The listing builds one solid part. Answer for the finished solid, in the listing's coordinates (mm). Face numbers are marked on the shaded views. Coordinates: 2 decimals unless noted, no trailing zeros. Write each loop counter-clockwise with the first axis right and the second up, starting at its lowest first coordinate (ties: lowest second). Pieces come first, ordered by that corner, then holes.
(1) Given P1, Ø4, axis at x = 2.5, y = -2, coming from the -Z side; P2, Ø1.5, axis at y = -5, z = 2.5, coming from the -X side, each flat-ended and moving along its own axis, determine where each tip first touches the part or whether it passes through.
(2) Straight lines are drawn through the part: line 1 (Y direction, x = 0, z = 1.25); line 2 (Y direction, x = -4, z = 0.25); line 3 (X direction, y = 0.5, z = 2.1). For each, find the intervals that lie inside material, in ascending order.
(3) The part is cut by section A-A on z = 1.25. Determine the outline of the cut face in (x, y), plus the area to 3 significant figures.
(4) The part is cut by section B-B on x = 0. Determine the outline of the cut face in (y, z).
(5) For a pull along Y with two mould halves and no side action, classify the marked faces 1, 2, 3 and 4 as +Y half, -Y half, draft (parallel to the pull), parting line (faces both ways), or undercut.
from build123d import *

# Parameters (mm, degrees)
SKIZZE2_W                            = 69.6667
SKIZZE2_H                            = 68.6667
SCHNITT_LINEAR_AUSTRAGEN1_DEPTH      = 10
SCHNITT_LINEAR_AUSTRAGEN1_DEPTH_BACK = 10


with BuildPart() as part:
    # Skizze1 → Rotation1 (revolve)
    with BuildSketch(Plane(origin=(0, 0, 0), x_dir=(0, 0, -1), z_dir=(1, 0, 0))):
        Polygon((-3, 6.5), (-3, 5), (-2.4585, 4.4585), (-0.5415, 4.4585), (0, 5), (0, 6.5), (-0.200961894, 7.25), (-2.799038106, 7.25), align=None)
    revolve(axis=Axis((0, 0, 0), (0, 0, 1)))

    # Skizze2 → Schnitt-Linear austragen1 (cut, two sides)
    with BuildSketch(Plane.XY) as schnitt_linear_austragen1_sk:
        with Locations((-1.75005, -1.16665)):
            Rectangle(SKIZZE2_W, SKIZZE2_H)
        Polygon((-6.5, -3.75277675), (0, -7.505553499), (6.5, -3.75277675), (6.5, 3.75277675), (0, 7.505553499), (-6.5, 3.75277675), align=None, mode=Mode.SUBTRACT)
    extrude(amount=SCHNITT_LINEAR_AUSTRAGEN1_DEPTH, mode=Mode.SUBTRACT)
    extrude(schnitt_linear_austragen1_sk.sketch, amount=-SCHNITT_LINEAR_AUSTRAGEN1_DEPTH_BACK, mode=Mode.SUBTRACT)


solid = part.part
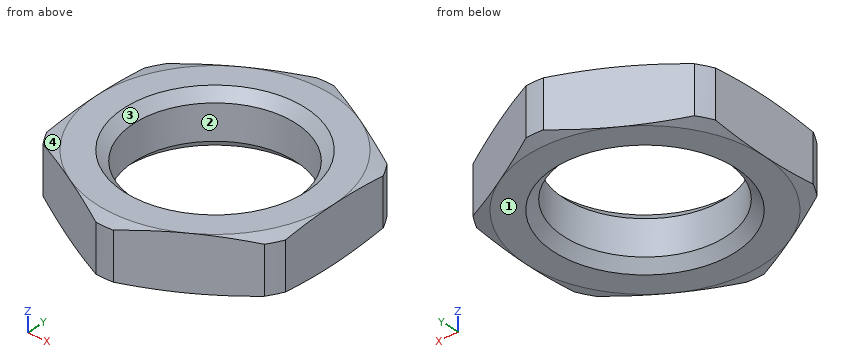
Model answer:
1. P1: stops at z = 0
1. P2: stops at x = -5.64
2. line 1: y = -7.25 to -4.46, 4.46 to 7.25
2. line 2: y = -5.2 to -2.56, 2.56 to 5.2
2. line 3: x = -6.5 to -4.43, 4.43 to 6.5
3. outline: (-6.5, -3.21) arc R7.25 ccw to (-6.03, -4.02) - (-0.47, -7.23) arc R7.25 ccw to (0.47, -7.23) - (6.03, -4.02) arc R7.25 ccw to (6.5, -3.21) - (6.5, 3.21) arc R7.25 ccw to (6.03, 4.02) - (0.47, 7.23) arc R7.25 ccw to (-0.47, 7.23) - (-6.03, 4.02) arc R7.25 ccw to (-6.5, 3.21) - close; hole circle Ø8.92 at (0, 0)
3. area: 83.2 mm2
4. outline: (-7.25, 0.2) - (-6.5, 0) - (-5, 0) - (-4.46, 0.54) - (-4.46, 2.46) - (-5, 3) - (-6.5, 3) - (-7.25, 2.8) - close; (4.46, 0.54) - (5, 0) - (6.5, 0) - (7.25, 0.2) - (7.25, 2.8) - (6.5, 3) - (5, 3) - (4.46, 2.46) - close
5. face 1: draft
5. face 2: undercut
5. face 3: undercut
5. face 4: -Y half
